Build history of the part. All positions in model axes, mm. Face numbers are marked on the shaded views. Coordinates: 2 decimals unless noted, no trailing zeros. Loops run counter-clockwise (first coordinate to the right, second up) from the corner with the lowest first, then second, coordinate; pieces in that order, holes last.
Item 1: Cut at B-B (x = 0). List the corners of the cut face in (y, z) (3 decimals), and give its area (3 significant figures).
Item 2: Flat gauge pins, fed straight in: pin 1 (3 mm diameter, centred on x = -17, y = -1, fed in from -Z); pin 2 (5 mm diameter, centred on y = -0.5, z = -3, fed in from +X); pin 3 (5 mm diameter, centred on x = -15, y = -1.5, fed in from +Z). Where does each tip first touch, or does it go through?
Item 3: Cut at D-D (z = 20.5). List the corners of the cut face in (x, y), and give its area (3 significant figures).
Item 4: Cut at C-C (y = 11.5). List the corners of the cut face in (x, z) (3 decimals).
Item 5: Mould opens along X. For the marked faces 1, 2, 3 and 4 say: released by +X, released by -X, zero draft, split by the parting line, or undercut.
Item 6: Cut at A-A (z = 0). List the corners of the cut face in (x, y) (3 decimals).
Item 7: Drill centre lines: line 1 along Z through (x, y) = (0, 12) (3 decimals); line 2 along Z through (x, y) = (0, -2); line 3 along Y through (x, z) = (-14, 15). Where is each one in solid material? Low to high.
from build123d import *

# Parameters (mm, degrees)
F0_R     = 25.4
F0_R_2   = 22.86
F1_DEPTH = 3.81
F2_DEPTH = 12.7
F3_R     = 25.4
F3_R_2   = 22.86
F3_R_3   = 13.1826
F4_DEPTH = 2.54
F3_R_4   = 9.525
F5_DEPTH = 17.78


with BuildPart() as f1:
    # F0 (on Front) → F1 (new body)
    with BuildSketch(Plane.XZ):
        Circle(F0_R)
        Circle(F0_R_2, mode=Mode.SUBTRACT)
    extrude(amount=F1_DEPTH)

    # F0 (on Front) → F2 (join)
    with BuildSketch(Plane.XZ):
        Circle(F0_R)
        Circle(F0_R_2, mode=Mode.SUBTRACT)
    extrude(amount=F2_DEPTH)

    # F3 (on face) → F4 (join)
    with BuildSketch(Plane(origin=(0, 0, 0), x_dir=(-1, 0, 0), z_dir=(0, 1, 0))):
        Circle(F3_R)
        Circle(F3_R_2, mode=Mode.SUBTRACT)
        Circle(F3_R_2)
        Circle(F3_R_3, mode=Mode.SUBTRACT)
    extrude(amount=F4_DEPTH)

    # F3 (on face) → F5 (join)
    with BuildSketch(Plane(origin=(0, 0, 0), x_dir=(-1, 0, 0), z_dir=(0, 1, 0))):
        Circle(F3_R_3)
        Circle(F3_R_4, mode=Mode.SUBTRACT)
    extrude(amount=F5_DEPTH)


solid = f1.part
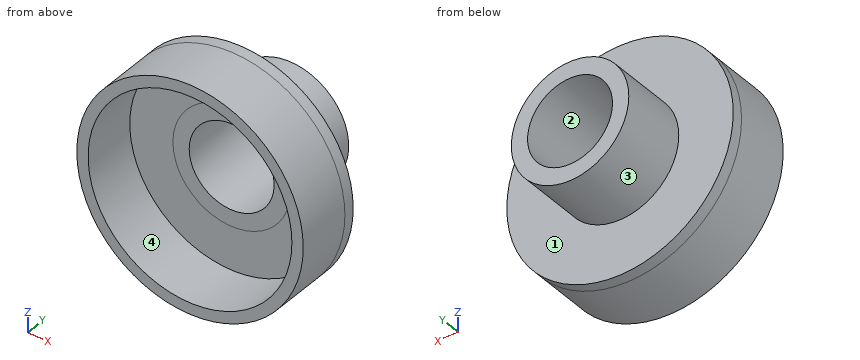
Filled sheet:
1. outline: (-12.7, -25.4) - (2.54, -25.4) - (2.54, -13.183) - (17.78, -13.183) - (17.78, -9.525) - (0, -9.525) - (0, -22.86) - (-12.7, -22.86) - close; (-12.7, 22.86) - (0, 22.86) - (0, 9.525) - (17.78, 9.525) - (17.78, 13.183) - (2.54, 13.183) - (2.54, 25.4) - (-12.7, 25.4) - close
1. area: 257 mm2
2. pin 1: stops at z = -20.12
2. pin 2: stops at x = 25.4
2. pin 3: stops at z = 22.11
3. outline: (-15, -12.7) - (-10.12, -12.7) - (-10.12, 0) - (10.12, 0) - (10.12, -12.7) - (15, -12.7) - (15, 2.54) - (-15, 2.54) - close
3. area: 200 mm2
4. outline: circle Ø26.365 at (0, 0); hole circle Ø19.05 at (0, 0)
5. face 1: zero draft
5. face 2: undercut
5. face 3: split by the parting line
5. face 4: undercut
6. outline: (-25.4, -12.7) - (-22.86, -12.7) - (-22.86, 0) - (-9.525, 0) - (-9.525, 17.78) - (-13.183, 17.78) - (-13.183, 2.54) - (-25.4, 2.54) - close; (9.525, 0) - (22.86, 0) - (22.86, -12.7) - (25.4, -12.7) - (25.4, 2.54) - (13.183, 2.54) - (13.183, 17.78) - (9.525, 17.78) - close
7. line 1: z = -13.183 to -9.525, 9.525 to 13.183
7. line 2: z = -25.4 to -22.86, 22.86 to 25.4
7. line 3: y = 0 to 2.54
